Answer from the drawing. Dimensions are ordinates in mm from the lowest x, y and z of the part. A direction names the side the tool comes from. Round coordinates to 2 decimals unless told otherwise and drop trailing zeros. Order: outer loops, then holes, each group sorted by start corner. A loop starts at its lowest first (then second) coordinate and runs counter-clockwise, first axis right, second up. Notation, with made-up numbers: (11.5, 87) - (52.5, 87) arc R12 ccw to (52.5, 102) - close; hole circle Ø8 at (73.5, 68). An arc over 180 degrees is marked (long way). One line per question, with ' | ' between items. Start each with the question number.
1) The part is cut by section D-D, the plane z = 12.5. Give the vertices of the cut face in (x, y).
2) The part is cut by section A-A, the plane x = 43.5. Give the vertices of the cut face in (y, z).
3) The mould has two halves that part along Z. Classify the marked faces 1, 2 and 3: pulls with the +Z half, pulls with the -Z half, needs draft (parallel to the pull), parting line crosses it, or undercut.
4) Flat-ended cylindrical pins translate along their axes: pin 1 (8 mm diameter, centred on y = 14.5, z = 6.5, fed in from -X); pin 2 (2.5 mm diameter, centred on x = 43.5, y = 17.5, fed in from -Z); pin 3 (1 mm diameter, centred on y = 4, z = 12.5, fed in from +X); pin 4 (3 mm diameter, centred on x = 19, z = 4, fed in from -Y). Find the tip coordinate at first contact, or state that the pin passes through.
5) The part is cut by section C-C, the plane y = 9.5. Give the vertices of the cut face in (x, z).
6) For the marked faces 4 and 5, determine the directions among +Z, -Z, +X, -X, +Y, -Y from which every point of the face is accessible in a straight line to the end or side of a thin tool.
7) Straight lines are drawn through the part: line 1 (Y direction, x = 43.5, z = 15.25); line 2 (Z direction, x = 30.5, y = 20); line 3 (X direction, y = 17.5, z = 15.25). For each, find the intervals that lie inside material, in ascending order. Write a range as from..to.
8) The part is cut by section B-B, the plane y = 17.5. Give the vertices of the cut face in (x, z).
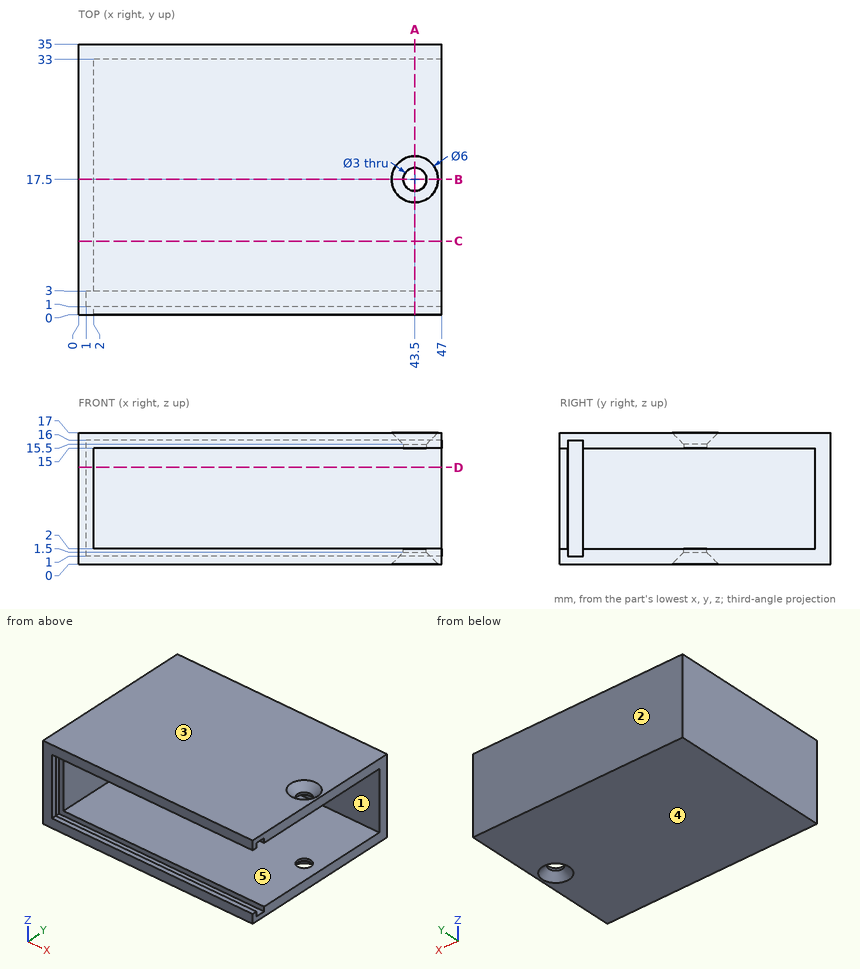
Values:
1) outline: (0, 0) - (2, 0) - (2, 1) - (1, 1) - (1, 3) - (2, 3) - (2, 33) - (47, 33) - (47, 35) - (0, 35) - close
2) outline: (0, 0) - (14.5, 0) - (16, 1.5) - (16, 2) - (3, 2) - (3, 1) - (1, 1) - (1, 2) - (0, 2) - close; (0, 15) - (1, 15) - (1, 16) - (3, 16) - (3, 15) - (16, 15) - (16, 15.5) - (14.5, 17) - (0, 17) - close; (19, 1.5) - (20.5, 0) - (35, 0) - (35, 17) - (20.5, 17) - (19, 15.5) - (19, 15) - (33, 15) - (33, 2) - (19, 2) - close
3) face 1: undercut | face 2: needs draft | face 3: pulls with the +Z half
4) pin 1: stops at x = 0 | pin 2: passes through | pin 3: stops at x = 2 | pin 4: stops at y = 33
5) outline: (0, 0) - (47, 0) - (47, 2) - (2, 2) - (2, 15) - (47, 15) - (47, 17) - (0, 17) - close
6) face 4: -Z, +X, -X, +Y, -Y | face 5: +X, -Y
7) line 1: y = 0..1, 3..16, 19..35 | line 2: z = 0..2, 15..17 | line 3: x = 0..42, 45..47
8) outline: (0, 0) - (40.5, 0) - (42, 1.5) - (42, 2) - (2, 2) - (2, 15) - (42, 15) - (42, 15.5) - (40.5, 17) - (0, 17) - close; (45, 1.5) - (46.5, 0) - (47, 0) - (47, 2) - (45, 2) - close; (45, 15) - (47, 15) - (47, 17) - (46.5, 17) - (45, 15.5) - close
